Read the model definition and answer for the solid it produces. Units are mm, in the model's axes. A direction names the side the tool comes from. Give positions to 0.01 mm unless a question says otherwise; leave off trailing zeros. Order: outer loops, then holes, each group sorted by start corner. A loop starts at its lowest first (then second) coordinate and runs counter-clockwise, first axis right, second up. Notation, with made-up numbers: (25.5, 15.25) - (58.5, 15.25) arc R23 cw to (58.5, 37.25) - close; hole circle Ø11 at (29.25, 54). An arc over 180 degrees is marked (long way). Write each question's results on one line, items separated by ' | '. Start each with the question number.
Q1. Find section A-A on y = -553. Give the vertices of the cut face in (x, z), and give its area (3 significant figures).
Q2. Find section C-C on y = -837. Give the vertices of the cut face in (x, z), and give its area (3 significant figures).
Q3. Find section B-B on z = -16.5. Give the vertices of the cut face in (x, y).
Q4. Find the intervals of material crossed by line 1 along X through (y, z) = (-222.5, -32); line 2 along X through (y, z) = (-385.5, -4); line 3 along Y through (x, z) = (-1662.5, -12), in increasing order. Write a range as from..to.
Q5. A tool of negligible diameter and unlimited length cuts with its end or side. For faces 4 (the face through (-1853.842, -580.105, -18.783)), 5 (the face through (-1767.862, -636.756, -18.783)), from which of +Z, -Z, +X, -X, +Y, -Y can it reach the whole face along a straight path? Write none if from no direction.
Q6. Find section D-D on x = -1690. Give the vertices of the cut face in (y, z).
Q7. For a pull along X with two mould halves and no side action, classify faces 1 (the face through (-1487, -336, 0)), 2 (the face through (-586.762, -580.105, -18.783)), 3 (the face through (-670.538, -636.756, -18.783)) as +X half, -X half, draft (parallel to the pull), parting line (faces both ways), or undercut.
Q8. Flat-ended cylindrical pins translate along their axes: P1, Ø6, axis at y = -772.5, z = -27.5, coming from the -X side; P2, Ø4, axis at x = -315.5, z = -15.5, coming from the -Y side; P3, Ø10, axis at y = -717, z = -8.5, coming from the -X side. Find the tip coordinate at first contact, or state that the pin passes through.
Autodesk Inventor part; units mm, degrees
ref_plane "YZ Plane" through (0, 0, 0) normal (1, 0, 0) x (0, 1, 0)
ref_plane "XZ Plane" through (0, 0, 0) normal (0, 1, 0) x (-1, 0, 0)
ref_plane "XY Plane" through (0, 0, 0) normal (0, 0, 1) x (1, 0, 0)
sketch "Sketch1" plane through (0, 0, 0) normal (0, 0, 1) x (1, 0, 0)
  line L0 (0, 0) -> (-2438.4, 0)
  line L1 (-38.1, 0) -> (-38.1, -1219.2)
  line L2 (0, -1219.2) -> (-2438.4, -1219.2)
  line L3 (-2400.3, 0) -> (-2400.3, -1219.2)
  line L4 (-2400.3, -1219.2) -> (-2400.3, -1144.1906)
  line L5 (-2400.3, -1144.1906) -> (-1291.8653, 0)
  line L6 (-1219.2, 0) -> (-1291.8653, 0)
  line L7 (-1219.2, -70.3945) -> (-2332.1053, -1219.2)
  line L8 (-2332.1053, -1219.2) -> (-2400.3, -1219.2)
  line L9 (-1219.2, -70.3945) -> (-106.2947, -1219.2)
  line L10 (-38.1, -1219.2) -> (-106.2947, -1219.2)
  line L11 (-38.1, -1219.2) -> (-38.1, -1144.1906)
  line L12 (-38.1, -1144.1906) -> (-1151.0053, 0)
  line L13 (-1219.2, 0) -> (-1151.0053, 0)
extrude "Extrusion1" add sketch "Sketch1" against normal blind 38.1 contours L12 L1 L2 L9 L7 L3 L5 L0
properties part number "48x2x4-2"
Working result:
1) outline: (-1827.58, -38.1) - (-1686.72, -38.1) - (-1686.72, 0) - (-1827.58, 0) - close; (-751.68, -38.1) - (-613.13, -38.1) - (-613.13, 0) - (-751.68, 0) - close | area: 10,600 mm²
2) outline: (-2102.71, -38.1) - (-1961.85, -38.1) - (-1961.85, 0) - (-2102.71, 0) - close; (-476.55, -38.1) - (-336.89, -38.1) - (-336.89, 0) - (-476.55, 0) - close | area: 10,700 mm²
3) outline: (-2400.3, -1219.2) - (-2332.11, -1219.2) - (-1219.2, -70.39) - (-106.29, -1219.2) - (-38.1, -1219.2) - (-38.1, -1144.19) - (-1151.01, 0) - (-1291.87, 0) - (-2400.3, -1144.19) - close
4) line 1: -1507.41..-1366.55, -1071.85..-934.59 | line 2: -1665.32..-1524.46, -913.94..-776.05 | line 3: -527.99..-382.59
5) face 4: +Z, -Z, -X, +Y | face 5: +Z, -Z, -Y
6) outline: (-556.38, -38.1) - (-410.98, -38.1) - (-410.98, 0) - (-556.38, 0) - close
7) face 1: draft | face 2: +X half | face 3: undercut
8) P1: x = -2043.13 | P2: y = -1005.31 | P3: x = -1991.3
